```python
from build123d import *

# Parameters (mm, degrees)
SKETCH1_W                         = 100
SKETCH1_H                         = 100
BOSS_EXTRUDE1_DEPTH               = 8.5
CUT_EXTRUDE1_DEPTH                = 142.676568281
SKETCH3_W                         = 8.5
SKETCH3_H                         = 8.5
BOSS_EXTRUDE2_DEPTH               = 6.5
TAP_DRILL_FOR_4_HELICOIL5_D       = 3.048
TAP_DRILL_FOR_4_HELICOIL5_DEPTH   = 5.69
TAP_DRILL_FOR_4_HELICOIL5_TIP     = 0.915711583
TAP_DRILL_FOR_4_HELICOIL5_4_D     = 3.048
TAP_DRILL_FOR_4_HELICOIL5_4_DEPTH = 5.69
TAP_DRILL_FOR_4_HELICOIL5_4_TIP   = 0.915711583
CUT_EXTRUDE2_DEPTH                = 7
CUT_EXTRUDE3_DEPTH                = 142.647449677
FILLET1_R                         = 1
FILLET2_R                         = 3.175
FILLET3_R                         = 0.79
TAP_DRILL_FOR_4_HELICOIL5_5_D     = 3.048
TAP_DRILL_FOR_4_HELICOIL5_5_DEPTH = 5.69
TAP_DRILL_FOR_4_HELICOIL5_5_TIP   = 0.915711583
TAP_DRILL_FOR_8_32_TAP1_D         = 3.4544
TAP_DRILL_FOR_8_32_TAP1_DEPTH     = 11.0998
TAP_DRILL_FOR_8_32_TAP1_TIP       = 1.037806461
SKETCH27_R                        = 2.8575
CUT_EXTRUDE4_DEPTH                = 2.032
SKETCH28_R                        = 2.286
CUT_EXTRUDE5_DEPTH                = 4.318
F_4_CLEARANCE_HOLE1_D             = 3.4544


with BuildPart() as part:
    # Sketch1 → Boss-Extrude1 (new body)
    with BuildSketch(Plane(origin=(0, 0, 0), x_dir=(1, 0, 0), z_dir=(0, 1, 0))):
        with Locations((50, 50)):
            Rectangle(SKETCH1_W, SKETCH1_H)
    extrude(amount=BOSS_EXTRUDE1_DEPTH)

    # Sketch2 → Cut-Extrude1 (cut, through all)
    with BuildSketch(Plane(origin=(0, 8.5, 0), x_dir=(1, 0, 0), z_dir=(0, 1, 0))):
        with BuildLine():
            Line((19.05, 100), (0, 100))
            Line((0, 100), (0, 83.590412453))
            Line((0, 83.590412453), (0, 80.95))
            Line((0, 80.95), (0, 80.554651577))
            ThreePointArc((0, 80.554651577), (1.825498063, 81.254538032), (1.5875, 83.19506403))
            Line((1.5875, 83.19506403), (1.5875, 98.4125))
            Line((1.5875, 98.4125), (16.80493597, 98.4125))
            ThreePointArc((16.80493597, 98.4125), (18.745461968, 98.174501937), (19.445348423, 100))
            Line((19.445348423, 100), (19.05, 100))
        make_face()
        with BuildLine():
            Line((80.95, 100), (80.554651577, 100))
            ThreePointArc((80.554651577, 100), (81.254538032, 98.174501937), (83.19506403, 98.4125))
            Line((83.19506403, 98.4125), (98.4125, 98.4125))
            Line((98.4125, 98.4125), (98.4125, 83.19506403))
            ThreePointArc((98.4125, 83.19506403), (98.174501937, 81.254538032), (100, 80.554651577))
            Line((100, 80.554651577), (100, 80.95))
            Line((100, 80.95), (100, 83.590412453))
            Line((100, 83.590412453), (100, 100))
            Line((100, 100), (80.95, 100))
        make_face()
        with BuildLine():
            Line((1.5875, 1.5875), (16.80493597, 1.5875))
            ThreePointArc((16.80493597, 1.5875), (18.745461968, 1.825498063), (19.445348423, 0))
            Line((19.445348423, 0), (19.05, 0))
            Line((19.05, 0), (0, 0))
            Line((0, 0), (0, 19.05))
            Line((0, 19.05), (0, 19.445348423))
            ThreePointArc((0, 19.445348423), (1.825498063, 18.745461968), (1.5875, 16.80493597))
            Line((1.5875, 16.80493597), (1.5875, 1.5875))
        make_face()
        with BuildLine():
            Line((98.4125, 1.5875), (83.19506403, 1.5875))
            ThreePointArc((83.19506403, 1.5875), (81.254538032, 1.825498063), (80.554651577, 0))
            Line((80.554651577, 0), (80.95, 0))
            Line((80.95, 0), (100, 0))
            Line((100, 0), (100, 19.05))
            Line((100, 19.05), (100, 19.445348423))
            ThreePointArc((100, 19.445348423), (98.174501937, 18.745461968), (98.4125, 16.80493597))
            Line((98.4125, 16.80493597), (98.4125, 1.5875))
        make_face()
    extrude(amount=-CUT_EXTRUDE1_DEPTH, mode=Mode.SUBTRACT)

    # Sketch3 → Boss-Extrude2 (add)
    with BuildSketch(Plane(origin=(0, 8.5, 0), x_dir=(1, 0, 0), z_dir=(0, 1, 0))):
        with Locations((4.25, 4.25)):
            Rectangle(SKETCH3_W, SKETCH3_H)
        with Locations((95.75, 4.25)):
            Rectangle(SKETCH3_W, SKETCH3_H)
        with Locations((95.75, 95.75)):
            Rectangle(SKETCH3_W, SKETCH3_H)
        with Locations((4.25, 95.75)):
            Rectangle(SKETCH3_W, SKETCH3_H)
    extrude(amount=BOSS_EXTRUDE2_DEPTH)

    # Tap Drill for _4 Helicoil5
    with Locations(Plane(origin=(0, 0, 0), x_dir=(-1, 0, 0), z_dir=(0, -1, 0))):
        with Locations((-87.465, 7.1375), (-90.005, 92.8625), (-13.805, 7.1375), (-9.995, 92.8625)):
            Hole(TAP_DRILL_FOR_4_HELICOIL5_D / 2, depth=TAP_DRILL_FOR_4_HELICOIL5_DEPTH)
            with Locations((0, 0, -(TAP_DRILL_FOR_4_HELICOIL5_DEPTH + TAP_DRILL_FOR_4_HELICOIL5_TIP / 2))):  # 118° drill point
                Cone(0, TAP_DRILL_FOR_4_HELICOIL5_D / 2, TAP_DRILL_FOR_4_HELICOIL5_TIP, mode=Mode.SUBTRACT)

    # Sketch18 → Tap Drill for _4 Helicoil5 2 (revolve, cut)
    with BuildSketch(Plane(origin=(1.5875, 4.5, -86.4125), x_dir=(0, 0, 1), z_dir=(0, 1, 0))):
        Polygon((0, 0), (0, 6.605711583), (1.524, 5.69), (1.524, 0), align=None)
    tap_drill_for_4_helicoil5_2 = revolve(axis=Axis((-4.7625, 4.5, -86.4125), (1, 0, 0)), mode=Mode.SUBTRACT)

    # Mirror1: Tap Drill for _4 Helicoil5 2 across plane
    add(tap_drill_for_4_helicoil5_2.mirror(Plane(origin=(0, 0, -50), x_dir=(1, 0, 0), z_dir=(0, 0, -1))), mode=Mode.SUBTRACT)

    # Mirror2: Tap Drill for _4 Helicoil5 2 across plane
    add(tap_drill_for_4_helicoil5_2.mirror(Plane.ZY.offset(-50)), mode=Mode.SUBTRACT)

    # Mirror2 copy 1 sketch → Mirror2 copy 1 (revolve, cut)
    with BuildSketch(Plane(origin=(98.4125, 4.5, -13.5875), x_dir=(0, 0, -1), z_dir=(0, 1, 0))):
        Polygon((0, 0), (0, 6.605711583), (1.524, 5.69), (1.524, 0), align=None)
    revolve(axis=Axis((104.7625, 4.5, -13.5875), (-1, 0, 0)), mode=Mode.SUBTRACT)

    # Sketch21 → Tap Drill for _4 Helicoil5 3 (revolve, cut)
    with BuildSketch(Plane(origin=(13.5875, 4.5, -98.4125), x_dir=(0, 1, 0), z_dir=(1, 0, 0))):
        Polygon((0, 0), (0, 6.605711583), (1.524, 5.69), (1.524, 0), align=None)
    tap_drill_for_4_helicoil5_3 = revolve(axis=Axis((13.5875, 4.5, -104.7625), (0, 0, 1)), mode=Mode.SUBTRACT)

    # Mirror3: Tap Drill for _4 Helicoil5 3 across plane
    add(tap_drill_for_4_helicoil5_3.mirror(Plane.ZY.offset(-50)), mode=Mode.SUBTRACT)

    # Tap Drill for _4 Helicoil5 4
    with Locations(Plane.XY.offset(-1.5875)):
        with Locations((90.7525, 4.5)):
            Hole(TAP_DRILL_FOR_4_HELICOIL5_4_D / 2, depth=TAP_DRILL_FOR_4_HELICOIL5_4_DEPTH)
            with Locations((0, 0, -(TAP_DRILL_FOR_4_HELICOIL5_4_DEPTH + TAP_DRILL_FOR_4_HELICOIL5_4_TIP / 2))):  # 118° drill point
                Cone(0, TAP_DRILL_FOR_4_HELICOIL5_4_D / 2, TAP_DRILL_FOR_4_HELICOIL5_4_TIP, mode=Mode.SUBTRACT)

    # Sketch22 → Cut-Extrude2 (cut)
    with BuildSketch(Plane.XZ):
        with BuildLine():
            Line((83.19506403, -9.5875), (88.825, -9.5875))
            ThreePointArc((88.825, -9.5875), (89.947532015, -10.052467985), (90.4125, -11.175))
            Line((90.4125, -11.175), (90.4125, -16.80493597))
            Line((90.4125, -16.80493597), (98.4125, -16.80493597))
            Line((98.4125, -16.80493597), (100, -16.80493597))
            Line((100, -16.80493597), (100, -83.19506403))
            Line((100, -83.19506403), (98.4125, -83.19506403))
            Line((98.4125, -83.19506403), (90.4125, -83.19506403))
            Line((90.4125, -83.19506403), (90.4125, -88.825))
            ThreePointArc((90.4125, -88.825), (89.947532015, -89.947532015), (88.825, -90.4125))
            Line((88.825, -90.4125), (83.19506403, -90.4125))
            Line((83.19506403, -90.4125), (83.19506403, -98.4125))
            Line((83.19506403, -98.4125), (83.19506403, -100))
            Line((83.19506403, -100), (16.80493597, -100))
            Line((16.80493597, -100), (16.80493597, -98.4125))
            Line((16.80493597, -98.4125), (16.80493597, -90.4125))
            Line((16.80493597, -90.4125), (11.175, -90.4125))
            ThreePointArc((11.175, -90.4125), (10.052467985, -89.947532015), (9.5875, -88.825))
            Line((9.5875, -88.825), (9.5875, -83.19506403))
            Line((9.5875, -83.19506403), (1.5875, -83.19506403))
            Line((1.5875, -83.19506403), (0, -83.19506403))
            Line((0, -83.19506403), (0, -16.80493597))
            Line((0, -16.80493597), (1.5875, -16.80493597))
            Line((1.5875, -16.80493597), (9.5875, -16.80493597))
            Line((9.5875, -16.80493597), (9.5875, -11.175))
            ThreePointArc((9.5875, -11.175), (10.052467985, -10.052467985), (11.175, -9.5875))
            Line((11.175, -9.5875), (16.80493597, -9.5875))
            Line((16.80493597, -9.5875), (16.80493597, -1.5875))
            Line((16.80493597, -1.5875), (16.80493597, 0))
            Line((16.80493597, 0), (83.19506403, 0))
            Line((83.19506403, 0), (83.19506403, -1.5875))
            Line((83.19506403, -1.5875), (83.19506403, -9.5875))
        make_face()
    extrude(amount=-CUT_EXTRUDE2_DEPTH, mode=Mode.SUBTRACT)

    # Sketch23 → Cut-Extrude3 (cut, through all)
    with BuildSketch(Plane.XZ.offset(-7)):
        with BuildLine():
            Line((11.175, -90.4125), (88.825, -90.4125))
            ThreePointArc((88.825, -90.4125), (89.947532015, -89.947532015), (90.4125, -88.825))
            Line((90.4125, -88.825), (90.4125, -11.175))
            ThreePointArc((90.4125, -11.175), (89.947532015, -10.052467985), (88.825, -9.5875))
            Line((88.825, -9.5875), (11.175, -9.5875))
            ThreePointArc((11.175, -9.5875), (10.052467985, -10.052467985), (9.5875, -11.175))
            Line((9.5875, -11.175), (9.5875, -88.825))
            ThreePointArc((9.5875, -88.825), (10.052467985, -89.947532015), (11.175, -90.4125))
        make_face()
    extrude(amount=-CUT_EXTRUDE3_DEPTH, mode=Mode.SUBTRACT)

    # Fillet1
    fillet1_edges = [part.edges().sort_by_distance(p)[0] for p in [
        (0, 11.75, 0),
        (0, 15, -4.25),
        (4.25, 15, 0),
        (8.5, 15, -4.25),
        (4.25, 15, -8.5),
        (100, 11.75, 0),
        (100, 15, -4.25),
        (95.75, 15, -8.5),
        (91.5, 15, -4.25),
        (95.75, 15, 0),
        (100, 11.75, -100),
        (95.75, 15, -100),
        (91.5, 15, -95.75),
        (95.75, 15, -91.5),
        (100, 15, -95.75),
        (0, 11.75, -100),
        (0, 15, -95.75),
        (4.25, 15, -91.5),
        (8.5, 15, -95.75),
        (4.25, 15, -100),
    ]]
    fillet(fillet1_edges, radius=FILLET1_R)

    # Fillet2
    fillet2_edges = [part.edges().sort_by_distance(p)[0] for p in [
        (9.5875, 3.5, -83.19506403),
        (90.4125, 3.5, -16.80493597),
        (90.4125, 3.5, -83.19506403),
        (83.19506403, 3.5, -90.4125),
        (16.80493597, 3.5, -90.4125),
        (9.5875, 3.5, -16.80493597),
        (16.80493597, 3.5, -9.5875),
        (83.19506403, 3.5, -9.5875),
    ]]
    fillet(fillet2_edges, radius=FILLET2_R)

    # Fillet3
    fillet3_edges = [part.edges().sort_by_distance(p)[0] for p in [
        (98.4125, 4.25, -98.4125),
        (1.5875, 4.25, -1.5875),
        (98.4125, 4.25, -1.5875),
        (1.5875, 4.25, -98.4125),
    ]]
    fillet(fillet3_edges, radius=FILLET3_R)

    # Tap Drill for _4 Helicoil5 5
    with Locations(Plane.XY.offset(-1.5875)):
        with Locations((8.3875, 4.5)):
            Hole(TAP_DRILL_FOR_4_HELICOIL5_5_D / 2, depth=TAP_DRILL_FOR_4_HELICOIL5_5_DEPTH)
            with Locations((0, 0, -(TAP_DRILL_FOR_4_HELICOIL5_5_DEPTH + TAP_DRILL_FOR_4_HELICOIL5_5_TIP / 2))):  # 118° drill point
                Cone(0, TAP_DRILL_FOR_4_HELICOIL5_5_D / 2, TAP_DRILL_FOR_4_HELICOIL5_5_TIP, mode=Mode.SUBTRACT)

    # Tap Drill for #8-32 Tap1
    with Locations(Plane(origin=(0, 15, 0), x_dir=(1, 0, 0), z_dir=(0, 1, 0))):
        with Locations((4.25, 95.75), (95.75, 4.25)):
            Hole(TAP_DRILL_FOR_8_32_TAP1_D / 2, depth=TAP_DRILL_FOR_8_32_TAP1_DEPTH)
            with Locations((0, 0, -(TAP_DRILL_FOR_8_32_TAP1_DEPTH + TAP_DRILL_FOR_8_32_TAP1_TIP / 2))):  # 118° drill point
                Cone(0, TAP_DRILL_FOR_8_32_TAP1_D / 2, TAP_DRILL_FOR_8_32_TAP1_TIP, mode=Mode.SUBTRACT)

    # Sketch27 → Cut-Extrude4 (cut)
    with BuildSketch(Plane(origin=(0, 15, 0), x_dir=(1, 0, 0), z_dir=(0, 1, 0))):
        with Locations(Location((95.75, 95.75, 0), (0, 0, 270))):
            Circle(SKETCH27_R)
        with Locations(Location((4.25, 4.25, 0), (0, 0, 270))):
            Circle(SKETCH27_R)
    extrude(amount=-CUT_EXTRUDE4_DEPTH, mode=Mode.SUBTRACT)

    # Sketch28 → Cut-Extrude5 (cut)
    with BuildSketch(Plane(origin=(0, 12.968, 0), x_dir=(1, 0, 0), z_dir=(0, 1, 0))):
        with Locations(Location((95.75, 95.75, 0), (0, 0, 270))):
            Circle(SKETCH28_R)
        with Locations(Location((4.25, 4.25, 0), (0, 0, 270))):
            Circle(SKETCH28_R)
    extrude(amount=-CUT_EXTRUDE5_DEPTH, mode=Mode.SUBTRACT)

    # #4 Clearance Hole1 (through all)
    with Locations(Plane(origin=(0, 8.65, 0), x_dir=(1, 0, 0), z_dir=(0, 1, 0))):
        with Locations((4.25, 4.25), (95.75, 95.75)):
            Hole(F_4_CLEARANCE_HOLE1_D / 2)


solid = part.part
```
Source: CAD feature listing. Evaluate the final solid. Frame: model axes, mm. A direction names the side the tool comes from. Round coordinates to 2 decimals unless told otherwise and drop trailing zeros. Loops run counter-clockwise (first coordinate to the right, second up) from the corner with the lowest first, then second, coordinate; pieces in that order, holes last. Notation, with made-up numbers: M 19,-35 L 68,-35 A18 cw 68,-25 Z; hole C 70,63.25 d1. An arc over 180 degrees is marked long. Put each result on its own line as item: value.
(1) Section B-B, the plane y = 10. Return loops of the section in (x, z), and give its area (3 significant figures).
Solutions:
outline: M 0,-99 A1 ccw 1,-100 L 8.5,-100 L 8.5,-91.5 L 0,-91.5 Z; M 0,-8.5 L 8.5,-8.5 L 8.5,0 L 1,0 A1 ccw 0,-1 Z; M 91.5,-100 L 99,-100 A1 ccw 100,-99 L 100,-91.5 L 91.5,-91.5 Z; M 91.5,-8.5 L 100,-8.5 L 100,-1 A1 ccw 99,0 L 91.5,0 Z; hole C 4.25,-4.25 d4.57; hole C 4.25,-95.75 d3.45; hole C 95.75,-95.75 d4.57; hole C 95.75,-4.25 d3.45
area: 237 mm²
(2) Pull-direction query (Z, two-part tool) for faces 1 (the face through (13.409, 4.305, -91.966)), 2 (the face through (15.85, 3.55, -91.32)), 3 (the face through (5, 11, 0)), 4 (the face through (96, 3, -83.195)); classes: released by +Z, released by -Z, zero draft, split by the parting line, or undercut.
Solutions:
face 1: released by -Z
face 2: undercut
face 3: released by +Z
face 4: undercut
(3) Access query for faces 5 (the face through (100, 11, -5)), 6 (the face through (96.608, 13.998, -93.024)), 7 (the face through (84.925, 4.17, -95.607)), 8 (the face through (9, 4, -98.412)), 9 (the face through (8.5, 11, -4)). Directions: +Z, -Z, +X, -X, +Y, -Y. A direction counts if a zero-diameter tool reaches every point of the face in a straight line with its end or side. Return the directions, or none.
Solutions:
face 5: +Z, -Z, +X, +Y, -Y
face 6: +Y
face 7: -Z
face 8: -Z, -X, -Y
face 9: +Z, -Z, +Y
(4) Ray query, line 1 (Z direction, x = 4, y = 4.5); line 2 (Z direction, x = 95.75, y = 6.25); line 3 (X direction, y = 9, z = -92.5). Return the intervals inside material, ascending. Write a range as [from, to].
Solutions:
line 1: [-98.41, -97.46], [-94.04, -87.94], [-84.89, -83.2], [-16.8, -15.11], [-12.06, -5.96], [-2.54, -1.59]
line 2: [-98.41, -97.48], [-94.02, -83.2], [-16.8, -5.98], [-2.52, -1.59]
line 3: [0, 8.5], [91.5, 100]
(5) Section C-C, the plane x = 63.5. Return loops of the section in (y, z), and give its area (3 significant figures).
Solutions:
outline: M 7,-100 L 8.5,-100 L 8.5,-90.41 L 7,-90.41 Z; M 7,-9.59 L 8.5,-9.59 L 8.5,0 L 7,0 Z
area: 28.8 mm²
(6) First-contact query: pin 1 (10 mm diameter, centred on x = 46.5, z = -11.5, fed in from -Y); pin 2 (2.5 mm diameter, centred on x = 86.41, y = 4.5, fed in from -Z); pin 3 (2.5 mm diameter, centred on y = 4.5, z = -13.59, fed in from +X); pin 4 (5 mm diameter, centred on y = 12, z = -30.5, fed in from -X). Flat tips, straight axial feed; report the tip coordinate or a pass-through.
Solutions:
pin 1: y = 7
pin 2: z = -92.56
pin 3: x = 92.56
pin 4: through
(7) Section A-A, the plane z = -37.5. Return loops of the section in (x, y), and give its area (3 significant figures).
Solutions:
outline: M 0,7 L 9.59,7 L 9.59,8.5 L 0,8.5 Z; M 90.41,7 L 100,7 L 100,8.5 L 90.41,8.5 Z
area: 28.8 mm²
